CAD build for the part. Positions are in the model's coordinates, mm. Coordinates: 2 decimals unless noted, no trailing zeros. Loops run counter-clockwise (first coordinate to the right, second up) from the corner with the lowest first, then second, coordinate; pieces in that order, holes last. Notation, with made-up numbers: (20, 55.25) -> (67, 55.25) arc R26 ccw to (67, 90.25) -> close; hole circle Ø1 at (36, 86). An arc over 180 degrees is marked (long way). Answer as CSV lines item,"result". Start each with the question number.
```python
from build123d import *

# Parameters (mm, degrees)
BOSS_EXTRUDE1_DEPTH = 9.525
BOSS_EXTRUDE2_DEPTH = 9.525
SKETCH4_W           = 63.5
SKETCH4_H           = 355.6
BOSS_EXTRUDE3_DEPTH = 9.525
SKETCH5_R           = 9.525
CUT_EXTRUDE1_DEPTH  = 648.271856043


with BuildPart() as part:
    # Sketch1 → Boss-Extrude1 (new body)
    with BuildSketch(Plane(origin=(0, 0, 0), x_dir=(1, 0, 0), z_dir=(0, 1, 0))):
        Polygon((461.512355724, 17.636671785), (558.8, 99.270698215), (558.8, 177.8), (228.6, 177.8), (228.6, -177.8), align=None)
    extrude(amount=BOSS_EXTRUDE1_DEPTH)

    # Sketch1_4 → Boss-Extrude2 (add)
    with BuildSketch(Plane(origin=(0, 0, 0), x_dir=(1, 0, 0), z_dir=(0, 1, 0))):
        Polygon((558.8, -177.8), (558.8, 99.270698215), (461.512355724, 17.636671785), (228.6, -177.8), align=None)
    extrude(amount=BOSS_EXTRUDE2_DEPTH)

    # Sketch4 → Boss-Extrude3 (add)
    with BuildSketch(Plane.XZ):
        with Locations((196.85, 0)):
            Rectangle(SKETCH4_W, SKETCH4_H)
        with Locations((590.55, 0)):
            Rectangle(SKETCH4_W, SKETCH4_H)
    extrude(amount=-BOSS_EXTRUDE3_DEPTH)

    # Sketch5 → Cut-Extrude1 (cut, through all)
    with BuildSketch(Plane.XZ):
        with Locations(Location((495.3, 0, 0), (0, 0, 270))):
            Circle(SKETCH5_R)
        with Locations(Location((292.1, 0, 0), (0, 0, 270))):
            Circle(SKETCH5_R)
        with Locations(Location((495.3, -95.25, 0), (0, 0, 270))):
            Circle(SKETCH5_R)
        with Locations(Location((495.3, 95.25, 0), (0, 0, 270))):
            Circle(SKETCH5_R)
    extrude(amount=-CUT_EXTRUDE1_DEPTH, mode=Mode.SUBTRACT)


solid = part.part
```
Q1. Probe probe 1 along X at (y, z) = (3, 0) (3 decimals); probe 2 along X at (y, z) = (2.75, -95.25) (3 decimals); probe 3 along X at (y, z) = (2.25, 7). List the from-to ranges inside material, lowest first. Write a range as from..to.
Q2. Saw through at C-C (x = 292.1). List the corners of the cut face in (y, z) (3 decimals).
Q3. Saw through at D-D (z = -95.25). List the corners of the cut face in (x, y) (3 decimals).
Q4. Saw through at A-A (z = 0). List the corners of the cut face in (x, y) (3 decimals), and give its area (3 significant figures).
Q5. Saw through at B-B (x = 495.3). List the corners of the cut face in (y, z) (3 decimals).
Q6. Two-plate mould, pull along Z, no slides. Class faces 1 (the cylindrical face through (301.544, 4.696, 1.24)), 2 (the flat face through (622.3, 5, -2)), 3 (the flat face through (390, 5, 177.8)): pulls with the +Z half, pulls with the -Z half, needs draft (parallel to the pull), parting line crosses it, or undercut.
Ans:
1,probe 1,"x = 165.1..282.575, 301.625..485.775, 504.825..622.3"
1,probe 2,"x = 165.1..485.775, 504.825..622.3"
1,probe 3,"x = 165.1..285.64, 298.56..488.84, 501.76..622.3"
2,outline,"(0, -177.8) -> (9.525, -177.8) -> (9.525, -9.525) -> (0, -9.525) -> close; (0, 9.525) -> (9.525, 9.525) -> (9.525, 177.8) -> (0, 177.8) -> close"
3,outline,"(165.1, 0) -> (485.775, 0) -> (485.775, 9.525) -> (165.1, 9.525) -> close; (504.825, 0) -> (622.3, 0) -> (622.3, 9.525) -> (504.825, 9.525) -> close"
4,outline,"(165.1, 0) -> (282.575, 0) -> (282.575, 9.525) -> (165.1, 9.525) -> close; (301.625, 0) -> (485.775, 0) -> (485.775, 9.525) -> (301.625, 9.525) -> close; (504.825, 0) -> (622.3, 0) -> (622.3, 9.525) -> (504.825, 9.525) -> close"
4,area,"3,990 mm²"
5,outline,"(0, -177.8) -> (9.525, -177.8) -> (9.525, -104.775) -> (0, -104.775) -> close; (0, -85.725) -> (9.525, -85.725) -> (9.525, -9.525) -> (0, -9.525) -> close; (0, 9.525) -> (9.525, 9.525) -> (9.525, 85.725) -> (0, 85.725) -> close; (0, 104.775) -> (9.525, 104.775) -> (9.525, 177.8) -> (0, 177.8) -> close"
6,face 1,"undercut"
6,face 2,"needs draft"
6,face 3,"pulls with the +Z half"
